The listing builds one solid part. Answer for the finished solid, in the listing's coordinates (mm). A direction names the side the tool comes from. Give positions to 0.01 mm unless a question says otherwise; leave off trailing zeros. Write each loop counter-clockwise with the first axis right and the second up, starting at its lowest first coordinate (ties: lowest second). Pieces come first, ordered by that corner, then holes. Notation, with made-up numbers: (74.25, 80.5) - (95.25, 80.5) arc R34 cw to (95.25, 119.5) - close; hole circle Ø7 at (65, 45.5). An arc over 180 degrees is marked (long way). One line per item, written item: value. Start each with the question number.
from build123d import *

# Parameters (mm, degrees)
EXTRUDE_2_DEPTH = 48
SKETCH_4_R      = 11
EXTRUDE_3_DEPTH = 2
SKETCH_5_R      = 2.5
EXTRUDE_4_DEPTH = 18
SKETCH_6_R      = 200
EXTRUDE_5_DEPTH = 4


with BuildPart() as part:
    # 草圖3 → 填料-伸長2 (new body)
    with BuildSketch(Plane(origin=(0, 0, 0), x_dir=(1, 0, 0), z_dir=(0, 1, 0))):
        Polygon((-21.15, 0), (-21.15, 15.5), (-15.5, 21.15), (0, 21.15), (15.5, 21.15), (21.15, 15.5), (21.15, 0), (21.15, -15.5), (15.5, -21.15), (0, -21.15), (-15.5, -21.15), (-21.15, -15.5), align=None)
    extrude(amount=EXTRUDE_2_DEPTH)

    # 草圖4 → 填料-伸長3 (add)
    with BuildSketch(Plane(origin=(0, 48, 0), x_dir=(1, 0, 0), z_dir=(0, 1, 0))):
        with Locations(Location((0, 0, 0), (0, 0, 270))):
            Circle(SKETCH_4_R)
    extrude(amount=EXTRUDE_3_DEPTH)

    # 草圖5 → 填料-伸長4 (add)
    with BuildSketch(Plane(origin=(0, 50, 0), x_dir=(1, 0, 0), z_dir=(0, 1, 0))):
        with Locations(Location((0, 0, 0), (0, 0, 270))):
            Circle(SKETCH_5_R)
    extrude(amount=EXTRUDE_4_DEPTH)

    # 草圖6 → 填料-伸長5 (add)
    with BuildSketch(Plane(origin=(0, 68, 0), x_dir=(1, 0, 0), z_dir=(0, 1, 0))):
        with Locations(Location((0, 0, 0), (0, 0, 270))):
            Circle(SKETCH_6_R)
    extrude(amount=EXTRUDE_5_DEPTH)


solid = part.part
Item 1: Each of these flat-tipped pins is pushed along its axis until it touches: pin 1 Ø15.5 at (y, z) = (24.5, -5.5) entering from +X; pin 2 Ø9.5 at (x, y) = (-1, 19.5) entering from +Z; pin 3 Ø25 at (y, z) = (16.5, 0.5) entering from -X. Where does it stop, or does it pass through?
Item 2: The mould has two halves that part along Y. Classify faces 1 (the cylindrical face through (-10.74, 48.99, -2.38)), 2 (the flat face through (0, 24, -21.15)), 3 (the flat face through (10, 48, 9)), 4 (the flat face through (3, 72, -3)): +Y half, -Y half, draft (parallel to the pull), parting line (faces both ways), or undercut.
Item 3: Find section A-A on y = 15. Determine the outline of the cut face in (x, z).
Item 4: Find section B-B on x = -44.5. Determine the outline of the cut face in (y, z).
Item 5: Find section C-C on z = -115. Determine the outline of the cut face in (x, y), plus the area to 3 significant figures.
Item 6: Straight lines are drawn through the part: line 1 along Y through (x, z) = (-180.5, 80); line 2 along X through (y, z) = (6.5, 1.5); line 3 along Z through (x, y) = (-18, 3.5). For each, find the intervals that lie inside material, in ascending order.
Item 7: Find section D-D on y = 59. Determine the outline of the cut face in (x, z), plus the area to 3 significant figures.
Item 8: For faces 5 (the flat face through (0, 24, 21.15)), 6 (the flat face through (-21.15, 24, 0)), 7 (the flat face through (21.15, 24, 0)), determine the directions among +Z, -Z, +X, -X, +Y, -Y from which every point of the face is accessible in a straight line to the end or side of a thin tool.
Values:
1. pin 1: x = 21.15
1. pin 2: z = 21.15
1. pin 3: x = -21.15
2. face 1: undercut
2. face 2: draft
2. face 3: undercut
2. face 4: +Y half
3. outline: (-21.15, -15.5) - (-15.5, -21.15) - (15.5, -21.15) - (21.15, -15.5) - (21.15, 15.5) - (15.5, 21.15) - (-15.5, 21.15) - (-21.15, 15.5) - close
4. outline: (68, -194.99) - (72, -194.99) - (72, 194.99) - (68, 194.99) - close
5. outline: (-163.63, 68) - (163.63, 68) - (163.63, 72) - (-163.63, 72) - close
5. area: 1,310 mm^2
6. line 1: 68 to 72
6. line 2: -21.15 to 21.15
6. line 3: -18.65 to 18.65
7. outline: circle Ø5 at (0, 0)
7. area: 19.6 mm^2
8. face 5: +Z, +X, -X, -Y
8. face 6: +Z, -Z, -X, -Y
8. face 7: +Z, -Z, +X, -Y
